```python
from build123d import *
from build123d.topology import SkipClean

# Parameters (mm, degrees)
LEFT_ARM_DEPTH                = 12.5
SKETCH2_R                     = 20
LEFT_BOSS_DEPTH               = 30
LEFT_HEX_DEPTH                = 233.486558751
LEFT_HEX_DEPTH_BACK           = 233.486558751
SKETCH3_R                     = 65
CENTRE_BOSS_DEPTH             = 35
SKETCH5_W                     = 25
SKETCH5_H                     = 40
RIGHT_ARM_DEPTH               = 180
SKETCH7_R                     = 30
RIGHT_BOSS_DEPTH              = 30
SKETCH8_R                     = 17.5
RIGHT_BOSS_HOLE_DEPTH         = 368.848119787
SKETCH9_R                     = 40
CENTRE_HOLE_DEPTH             = 369.764476639
SKETCH10_R                    = 27.5
CENTRE_BLOB_DEPTH             = 35
CENTRE_BEAM_REACH             = 222.573
SKETCH11_W                    = 50
SKETCH11_H                    = 30
CENTRE_BEAM_DIRECTION_2_REACH = 222.573
SKETCH12_R                    = 20
CUT_EXTRUDE4_DEPTH            = 5
F_1_4_20_TAPPED_HOLE1_D       = 5.1054
CIRPATTERN1_COUNT             = 8
CUT_OUT_DEPTH                 = 10
FILLET1_R                     = 10
FILLET1_OF_MIRROR2_R          = 10


with BuildPart() as part:
    # Sketch1 → LEFT_ARM (new, symmetric)
    with BuildSketch(Plane.XY):
        with BuildLine():
            Line((-6, 19.078784028), (130.5, 62.006048092))
            ThreePointArc((130.5, 62.006048092), (215, 0), (130.5, -62.006048092))
            Line((130.5, -62.006048092), (-6, -19.078784028))
            ThreePointArc((-6, -19.078784028), (-20, 0), (-6, 19.078784028))
        make_face()
    extrude(amount=LEFT_ARM_DEPTH, both=True)

    # Sketch2 → LEFT_Boss (add, symmetric)
    with SkipClean():  # the faces are left unmerged after this step: merging them gives an invalid solid
        with BuildSketch(Plane.XY):
            Circle(SKETCH2_R)
        extrude(amount=LEFT_BOSS_DEPTH, both=True)

    # Sketch4 → LEFT_Hex (cut, two sides: drawn at the far end of the back side and taken through both)
    with SkipClean():  # the faces are left unmerged after this step: merging them gives an invalid solid
        with BuildSketch(Plane.XY.offset(30).offset(-LEFT_HEX_DEPTH_BACK)):
            Polygon((14.43375673, 0), (7.216878365, 12.5), (-7.216878365, 12.5), (-14.43375673, 0), (-7.216878365, -12.5), (7.216878365, -12.5), align=None)
        extrude(amount=LEFT_HEX_DEPTH + LEFT_HEX_DEPTH_BACK, mode=Mode.SUBTRACT)

    # Sketch3 → CENTRE_Boss (add, symmetric)
    with SkipClean():  # the faces are left unmerged after this step: merging them gives an invalid solid
        with BuildSketch(Plane.XY):
            with Locations((150, 0)):
                Circle(SKETCH3_R)
        extrude(amount=CENTRE_BOSS_DEPTH, both=True)

    # Sketch5 → RIGHT_ARM (add)
    with SkipClean():  # the faces are left unmerged after this step: merging them gives an invalid solid
        with BuildSketch(Plane(origin=(139.951905284, -37.5, 0), x_dir=(0, 0, -1), z_dir=(0.9659258262890681, -0.25881904510252135, 0))):
            with Locations((0, 38.822856765)):
                Rectangle(SKETCH5_W, SKETCH5_H)
        extrude(amount=RIGHT_ARM_DEPTH)

    # Sketch7 → RIGHT_Boss (add, symmetric)
    with SkipClean():  # the faces are left unmerged after this step: merging them gives an invalid solid
        with BuildSketch(Plane.XY):
            with Locations((323.866648732, -46.587428118)):
                Circle(SKETCH7_R)
        extrude(amount=RIGHT_BOSS_DEPTH, both=True)
    add(part.part.scale(1), mode=Mode.REPLACE)  # the faces are merged on a copy

    # Sketch8 → RIGHT_Boss_Hole (cut, through all)
    with BuildSketch(Plane.XY.offset(30)):
        with Locations((323.866648732, -46.587428118)):
            Circle(SKETCH8_R)
    extrude(amount=-RIGHT_BOSS_HOLE_DEPTH, mode=Mode.SUBTRACT)

    # Sketch9 → CENTRE_Hole (cut, through all)
    with BuildSketch(Plane.XY.offset(35)):
        with Locations((150, 0)):
            Circle(SKETCH9_R)
    extrude(amount=-CENTRE_HOLE_DEPTH, mode=Mode.SUBTRACT)

    # Sketch10 → CENTRE_Blob (add, symmetric)
    with SkipClean():  # the faces are left unmerged after this step: merging them gives an invalid solid
        with BuildSketch(Plane.XY):
            with Locations((174.148145657, -6.470476128)):
                Circle(SKETCH10_R)
        extrude(amount=CENTRE_BLOB_DEPTH, both=True)

    # Sketch11 → CENTRE_Beam (add, up to next)
    with BuildSketch(Plane(origin=(150, 0, 0), x_dir=(0, 0, -1), z_dir=(1, 0, 0)), mode=Mode.PRIVATE) as centre_beam_sk1:
        Rectangle(SKETCH11_W, SKETCH11_H)
    centre_beam_tool1 = extrude(centre_beam_sk1.sketch, amount=CENTRE_BEAM_REACH, mode=Mode.PRIVATE) - part.part
    add(centre_beam_tool1.solids().sort_by_distance((150, 0, 0))[0])

    # Sketch11 → CENTRE_Beam direction 2 (add, up to next)
    with BuildSketch(Plane(origin=(150, 0, 0), x_dir=(0, 0, -1), z_dir=(1, 0, 0)), mode=Mode.PRIVATE) as centre_beam_direction_2_sk1:
        Rectangle(SKETCH11_W, SKETCH11_H)
    centre_beam_direction_2_tool1 = extrude(centre_beam_direction_2_sk1.sketch, amount=-CENTRE_BEAM_DIRECTION_2_REACH, mode=Mode.PRIVATE) - part.part
    add(centre_beam_direction_2_tool1.solids().sort_by_distance((150, 0, 0))[0])

    # Sketch12 → Cut-Extrude4 (cut)
    with BuildSketch(Plane.XY.offset(35)):
        with Locations((174.148145657, -6.470476128)):
            Circle(SKETCH12_R)
    cut_extrude4 = extrude(amount=-CUT_EXTRUDE4_DEPTH, mode=Mode.SUBTRACT)

    # 1/4-20 Tapped Hole1 (through all)
    with Locations(Plane.XY.offset(30)):
        with Locations((159.659258263, -2.588190451)):
            f_1_4_20_tapped_hole1 = Hole(F_1_4_20_TAPPED_HOLE1_D / 2)

    # CirPattern1: 1/4-20 Tapped Hole1 ×8 about axis
    cirpattern1_axis = Axis((174.148145657, -6.470476128, 0), (0, 0, 1))
    for i in range(1, CIRPATTERN1_COUNT):
        add(f_1_4_20_tapped_hole1.rotate(cirpattern1_axis, i * 360 / CIRPATTERN1_COUNT), mode=Mode.SUBTRACT)

    # Mirror1: Cut-Extrude4 across plane
    add(cut_extrude4.mirror(Plane.XY), mode=Mode.SUBTRACT)

    # Sketch15 → Cut_OUT (cut)
    with BuildSketch(Plane.XY.offset(12.5)):
        with BuildLine():
            Line((84.858453972, 37.169597537), (23.981475126, 18.024673388))
            ThreePointArc((23.981475126, 18.024673388), (30, 0), (23.981475126, -18.024673388))
            Line((23.981475126, -18.024673388), (84.858453972, -37.169597537))
            ThreePointArc((84.858453972, -37.169597537), (75, 0), (84.858453972, 37.169597537))
        make_face()
    cut_out = extrude(amount=-CUT_OUT_DEPTH, mode=Mode.SUBTRACT)

    # Fillet1
    fillet1_edges = [part.edges().sort_by_distance(p)[0] for p in [
        (23.981475126, -18.024673388, 7.5),
        (23.981475126, 18.024673388, 7.5),
        (84.858453972, 37.169597537, 7.5),
        (84.858453972, -37.169597537, 7.5),
    ]]
    fillet(fillet1_edges, radius=FILLET1_R)

    # Mirror2: Cut_OUT across plane
    with SkipClean():  # the faces are left unmerged after this step: merging them gives an invalid solid
        add(cut_out.mirror(Plane.XY), mode=Mode.SUBTRACT)

    # Fillet1 of Mirror2
    fillet1_of_mirror2_edges = [part.edges().sort_by_distance(p)[0] for p in [
        (23.981475126, -18.024673388, -7.5),
        (23.981475126, 18.024673388, -7.5),
        (84.858453972, 37.169597537, -7.5),
        (84.858453972, -37.169597537, -7.5),
    ]]
    fillet(fillet1_of_mirror2_edges, radius=FILLET1_OF_MIRROR2_R)


solid = part.part
```
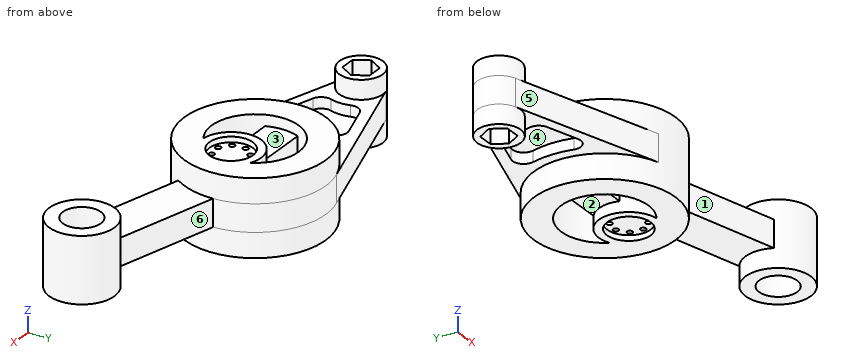
CAD build for the part. Positions are in the model's coordinates, mm. Face numbers are marked on the shaded views. A direction names the side the tool comes from. Give positions to 0.01 mm unless a question says otherwise; leave off trailing zeros. Loops run counter-clockwise (first coordinate to the right, second up) from the corner with the lowest first, then second, coordinate; pieces in that order, holes last. Notation, with made-up numbers: (77, 23) -> (128, 23) arc R23 ccw to (128, 49) -> close; hole circle Ø11 at (-28.75, 46). An arc over 180 degrees is marked (long way). Use a Markdown table: item, result.
1. Which spindle directions (+Z, -Z, +X, -X, +Y, -Y) get a long thin tool onto all of the face, cutting with end or side? Do the marked faces 1, 2 and 3. Say none if no direction does.
Check result:
| item | result |
|---|---|
| face 1 | +Z, -Z, -Y |
| face 2 | -Z |
| face 3 | +Z |
2. Wall check: L1, parallel to X at y = -31, z = -28.5; L2, parallel to X at y = -50, z = -17; L3, parallel to X at y = -9.5, z = -31. Give the ranges that are in metal, low to high. Write a range as [from, to].
Check result:
| item | result |
|---|---|
| L1 | x = [92.87, 124.72], [161.72, 207.13], [298.23, 315.91], [331.82, 349.5] |
| L2 | x = [108.47, 191.53], [294.06, 306.7], [341.03, 353.67] |
| L3 | x = [85.7, 111.14], [146.82, 154.38], [193.92, 214.3] |
3. Slice it at D-D (x = 0). List the corners of the cut face in (y, z), plus the area to 3 significant figures.
Check result:
| item | result |
|---|---|
| outline | (-20.97, -12.5) -> (-20, -12.5) -> (-20, -30) -> (-12.5, -30) -> (-12.5, 30) -> (-20, 30) -> (-20, 12.5) -> (-20.97, 12.5) -> close; (12.5, -30) -> (20, -30) -> (20, -12.5) -> (20.97, -12.5) -> (20.97, 12.5) -> (20, 12.5) -> (20, 30) -> (12.5, 30) -> close |
| area | 948 mm^2 |
4. Slice it at A-A (x = 324). List the corners of the cut face in (y, z), plus the area to 3 significant figures.
Check result:
| item | result |
|---|---|
| outline | (-76.59, -30) -> (-64.09, -30) -> (-64.09, 30) -> (-76.59, 30) -> close; (-29.09, -30) -> (-16.59, -30) -> (-16.59, 30) -> (-29.09, 30) -> close |
| area | 1,500 mm^2 |
5. Slice it at C-C (z = -20). Give the number of separate pieces and of enclosed holes in the cut face, plus the area to 3 significant figures.
Check result:
| item | result |
|---|---|
| separate pieces | 3 |
| enclosed holes | 12 |
| area | 13,600 mm^2 |
6. Flat gauge pins, fed straight in: pin 1 (12 mm diameter, centred on x = 128.5, z = 3, fed in from +Y); pin 2 (5 mm diameter, centred on y = -20.5, z = 9.5, fed in from -X); pin 3 (16 mm diameter, centred on x = -2, z = -2, fed in from +Y). Where does each tip first touch, or does it go through?
Check result:
| item | result |
|---|---|
| pin 1 | stops at y = 63.12 |
| pin 2 | stops at x = -8.72 |
| pin 3 | stops at y = 22.85 |
7. Mould opens along Y. For the marked faces 4, 5 and 6 say: pulls with the +Y half, pulls with the -Y half, needs draft (parallel to the pull), parting line crosses it, or undercut.
Check result:
| item | result |
|---|---|
| face 4 | undercut |
| face 5 | pulls with the -Y half |
| face 6 | pulls with the +Y half |
8. Slice it at B-B (y = -51.5). List the corners of the cut face in (x, z), plus the area to 3 significant figures.
Check result:
| item | result |
|---|---|
| outline | (97.09, -12.5) -> (110.34, -12.5) -> (110.34, -35) -> (189.66, -35) -> (189.66, 35) -> (110.34, 35) -> (110.34, 12.5) -> (97.09, 12.5) -> close; (264.93, -12.5) -> (294.27, -12.5) -> (294.27, -30) -> (307.07, -30) -> (307.07, 30) -> (294.27, 30) -> (294.27, 12.5) -> (264.93, 12.5) -> close; (340.66, -30) -> (353.46, -30) -> (353.46, 30) -> (340.66, 30) -> close |
| area | 8,150 mm^2 |
